For this review, take the finished solid that the model builds, in its own axes (mm). Round coordinates to 2 decimals unless told otherwise and drop trailing zeros. Loops run counter-clockwise (first coordinate to the right, second up) from the corner with the lowest first, then second, coordinate; pieces in that order, holes last.
1) Insertion check: pin 1 (5 mm diameter, centred on x = 1.5, y = 60.5, fed in from +Z); pin 2 (1.4 mm diameter, centred on x = 0, z = 17.9, fed in from +Y); pin 3 (3 mm diameter, centred on x = 0, z = -14.5, fed in from -Y). Each pin has a flat end and moves straight along its axis. Give the tip position at first contact, or say it passes through.
2) Wall thickness on L1, parallel to X at y = 11.9, z = -17.9; L2, parallel to X at y = 260, z = 0; L3, parallel to Y at x = 1.5, z = 15.5: over which ranges is each line inside the solid? List them lowest first.
3) Mouldability with a two-part tool opening along Y and no side actions: class faces 1 (the flat face through (-2, 0, 2)), 2 (the cylindrical face through (-5.37, 187.98, -1.19)), 3 (the flat face through (-2.4, 336.288, -0.1)), 4 (the cylindrical face through (-3.905, 17.983, -0.867)) as pulls with the +Y half, pulls with the -Y half, needs draft (parallel to the pull), parting line crosses it, or undercut.
4) Take a section at A-A (y = 113.5). State the section outline as (x, z) points.
```python
from build123d import *

# Parameters (mm, degrees)
SWEEP3_PROFILE_R         = 4
SWEEP4_PROFILE_R         = 5.5
SKETCH45_R               = 2.25
CUT_EXTRUDE2_DEPTH       = 337.377466094
SWEEP5_PROFILE_R         = 1
SWEEP6_PROFILE_R         = 1
SKETCH72_W               = 4.5
SKETCH72_H               = 20
CUT_EXTRUDE6_DEPTH       = 20
BOSS_EXTRUDE1_DEPTH      = 2.5
BOSS_EXTRUDE1_DEPTH_BACK = 2.5
BOSS_EXTRUDE3_DEPTH      = 2.5
BOSS_EXTRUDE3_DEPTH_BACK = 2.5
SKETCH76_4_W             = 16.5
SKETCH76_4_H             = 1.4
SKETCH77_R               = 0.612238256
CUT_EXTRUDE7_DEPTH       = 20
FILLET1_R                = 0.5


with BuildPart() as part:
    # Sweep3: sweep along a path in Sketch31
    with BuildLine(Plane.XY) as sweep3_path:
        Line((0, 0), (0, 35.470165431))
    # Sweep3 profile (on start of the path) → Sweep3 (sweep)
    with BuildSketch(Plane.ZX):
        Circle(SWEEP3_PROFILE_R)
    sweep(path=sweep3_path.line)

    # Sweep4: sweep along a path in Sketch38
    with BuildLine(Plane.XY) as sweep4_path:
        Line((0, 35.470165431), (0, 336.287525335))
    # Sweep4 profile (on start of the path) → Sweep4 (sweep)
    with BuildSketch(Plane.ZX.offset(35.470165431)):
        Circle(SWEEP4_PROFILE_R)
    sweep(path=sweep4_path.line)

    # Sketch45 → Cut-Extrude2 (cut, through all)
    with BuildSketch(Plane(origin=(0, 0, 0), x_dir=(1, 0, 0), z_dir=(0, 1, 0))):
        with Locations(Location((0, 0, 0), (0, 0, 270))):
            Circle(SKETCH45_R)
    extrude(amount=CUT_EXTRUDE2_DEPTH, mode=Mode.SUBTRACT)

    # Sweep5: sweep along a curve in space
    with BuildLine() as sweep5_path:
        Line((4, 336.287525335, 5.558e-06), (4, 337.787525335, 5.558e-06))
    # Sweep5 profile (on start of the path) → Sweep5 (sweep)
    with BuildSketch(Plane(origin=(4, 336.287525335, 5.558e-06), x_dir=(0, 0, 1), z_dir=(0, 1, 0))):
        Circle(SWEEP5_PROFILE_R)
    sweep(path=sweep5_path.line)

    # Sweep6: sweep along a curve in space
    with BuildLine() as sweep6_path:
        Line((-4, 336.287525335, 9.31e-07), (-4, 337.787525335, 9.31e-07))
    # Sweep6 profile (on start of the path) → Sweep6 (sweep)
    with BuildSketch(Plane(origin=(-4, 336.287525335, 9.31e-07), x_dir=(0, 0, 1), z_dir=(0, 1, 0))):
        Circle(SWEEP6_PROFILE_R)
    sweep(path=sweep6_path.line)

    # Sketch72 → Cut-Extrude6 (cut)
    with BuildSketch(Plane(origin=(0, 0, 0), x_dir=(0, 0, -1), z_dir=(1, 0, 0))):
        with Locations((-0.068000409, 19.236124066)):
            Rectangle(SKETCH72_W, SKETCH72_H)
    extrude(amount=CUT_EXTRUDE6_DEPTH, mode=Mode.SUBTRACT)

    # Sketch76 → Boss-Extrude1 (add, two sides: drawn at the far end of the back side and taken through both)
    with BuildSketch(Plane(origin=(0, 0, 0), x_dir=(0, 0, -1), z_dir=(1, 0, 0)).offset(-BOSS_EXTRUDE1_DEPTH_BACK)):
        Polygon((-3, 12.070165431), (-3, 12.770165431), (-19.5, 12.770165431), (-19.5, 12.370165431), (-19.5, 11.370165431), (-3, 11.370165431), align=None)
    extrude(amount=BOSS_EXTRUDE1_DEPTH + BOSS_EXTRUDE1_DEPTH_BACK)

    # Sketch76_4 → Boss-Extrude3 (add, two sides: drawn at the far end of the back side and taken through both)
    with BuildSketch(Plane(origin=(0, 0, 0), x_dir=(0, 0, -1), z_dir=(1, 0, 0)).offset(-BOSS_EXTRUDE3_DEPTH_BACK)):
        with Locations((11.25, 12.070165431)):
            Rectangle(SKETCH76_4_W, SKETCH76_4_H)
    extrude(amount=BOSS_EXTRUDE3_DEPTH + BOSS_EXTRUDE3_DEPTH_BACK)

    # Sketch77 → Cut-Extrude7 (cut)
    with BuildSketch(Plane(origin=(0, 0, 0), x_dir=(1, 0, 0), z_dir=(0, 1, 0))):
        with Locations(Location((0, 17.9, 0), (0, 0, 90))):
            Circle(SKETCH77_R)
        with Locations(Location((0, -17.9, 0), (0, 0, 90))):
            Circle(SKETCH77_R)
    extrude(amount=CUT_EXTRUDE7_DEPTH, mode=Mode.SUBTRACT)

    # Fillet1
    fillet1_edges = [part.edges().sort_by_distance(p)[0] for p in [
        (0, 12.770165431, 19.5),
        (2.5, 12.770165431, 11.3112495),
        (-2.5, 11.370165431, 11.3112495),
        (0, 11.370165431, 19.5),
        (2.5, 12.070165431, 19.5),
        (-2.5, 12.770165431, 11.3112495),
        (2.5, 11.370165431, 11.3112495),
        (0, 11.370165431, -19.5),
        (2.5, 11.370165431, -11.3112495),
        (2.5, 12.770165431, -11.3112495),
        (0, 12.770165431, -19.5),
        (-2.5, 12.770165431, -11.3112495),
        (-2.5, 11.370165431, -11.3112495),
        (2.5, 12.070165431, -19.5),
    ]]
    fillet(fillet1_edges, radius=FILLET1_R)


solid = part.part
```
Response:
1. pin 1: stops at z = 5.5
1. pin 2: stops at y = 12.77
1. pin 3: stops at y = 11.37
2. L1: x = -2.5 to -0.61, 0.61 to 2.5
2. L2: x = -5.5 to -2.25, 2.25 to 5.5
2. L3: y = 11.37 to 12.77
3. face 1: pulls with the -Y half
3. face 2: needs draft
3. face 3: pulls with the +Y half
3. face 4: undercut
4. outline: circle Ø11 at (0, 0); hole circle Ø4.5 at (0, 0)
